Could you check a few things on this model? Use its own coordinates, in mm. Face numbers are marked on the shaded views. A direction names the side the tool comes from. Give positions to 0.01 mm unless a question says otherwise; leave off trailing zeros. Order: outer loops, then holes, each group sorted by start corner. A loop starts at its lowest first (then second) coordinate and runs counter-clockwise, first axis right, second up. Notation, with made-up numbers: M 41,-6 L 69,-6 A28 ccw 69,22 Z; hole C -6.5,-36.5 d3. An arc over 180 degrees is marked long. Use a Markdown table: item, result. Add a question column.
Item 1: Suppose I cut it at C-C on z = 37. Write out the boundary of the cut face in (x, y), plus the area to 3 significant figures.
Item 2: If we mould it in two halves opening along Z, with no side actions, what happens to the marked faces 3, 4 and 5? For each: released by +Z, released by -Z, zero draft, split by the parting line, or undercut.
Item 3: Suppose I cut it at B-B on y = 15. Write out the boundary of the cut face in (x, z), plus the area to 3 significant figures.
Item 4: If I drill on L1, parallel to Z at x = 46.5, y = 12.5; L2, parallel to X at y = 3.5, z = 52; L3, parallel to X at y = 7.5, z = 57.5, over which ranges is the centre line in solid material (lowest first)? Write a range as from..to.
Item 5: Suppose I cut it at A-A on x = 20. Write out the boundary of the cut face in (y, z).
Item 6: For the marked faces 1 and 2, which set-ups out of +Z, -Z, +X, -X, +Y, -Y let a thin tool reach every point of the face, with its end or its side?
Item 7: I'm going to push a flat-ended pin straight in: pin 1 Ø6 at (y, z) = (5, 29.5) entering from +X. Where does the tip first touch, or does it pass through?
from build123d import *

# Parameters (mm, degrees)
BOX_W        = 60
BOX_H        = 20
BOX_DEPTH    = 15
BOX001_W     = 15
BOX001_H     = 20
BOX001_DEPTH = 70
BOX002_W     = 60
BOX002_H     = 20
BOX002_DEPTH = 15
FILLET_R     = 5


with BuildPart() as cube:
    # Box → Box (new body)
    with BuildSketch(Plane.XY):
        with Locations((30, 10)):
            Rectangle(BOX_W, BOX_H)
    extrude(amount=BOX_DEPTH)


with BuildPart() as cube001:
    # Box001 → Box001 (new body)
    with BuildSketch(Plane.XY):
        with Locations((7.5, 10)):
            Rectangle(BOX001_W, BOX001_H)
    extrude(amount=BOX001_DEPTH)


with BuildPart() as fillet_body:
    # Box002 → Box002 (new body)
    with BuildSketch(Plane.XY.offset(55)):
        with Locations((30, 10)):
            Rectangle(BOX002_W, BOX002_H)
    extrude(amount=BOX002_DEPTH)

    # Fusion: union Cube, Cube001
    add(cube.part)
    add(cube001.part)

    # Fillet
    fillet_edges = [fillet_body.edges().sort_by_distance(p)[0] for p in [
        (0, 10, 70),
        (60, 10, 70),
        (0, 10, 0),
        (60, 10, 55),
        (60, 10, 15),
        (60, 10, 0),
    ]]
    fillet(fillet_edges, radius=FILLET_R)


solid = fillet_body.part
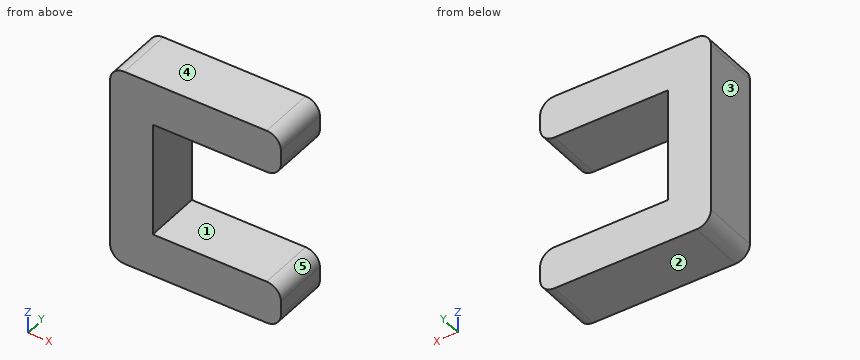
Findings below:
| question | item | result |
|---|---|---|
| 1 | outline | M 0,0 L 15,0 L 15,20 L 0,20 Z |
| 1 | area | 300 mm^2 |
| 2 | face 3 | zero draft |
| 2 | face 4 | released by +Z |
| 2 | face 5 | undercut |
| 3 | outline | M 0,5 A5 ccw 5,0 L 55,0 A5 ccw 60,5 L 60,10 A5 ccw 55,15 L 15,15 L 15,55 L 55,55 A5 ccw 60,60 L 60,65 A5 ccw 55,70 L 5,70 A5 ccw 0,65 Z |
| 3 | area | 2,370 mm^2 |
| 4 | L1 | z = 0..15, 55..70 |
| 4 | L2 | x = 0..15 |
| 4 | L3 | x = 0..59.33 |
| 5 | outline | M 0,0 L 20,0 L 20,15 L 0,15 Z; M 0,55 L 20,55 L 20,70 L 0,70 Z |
| 6 | face 1 | +X, +Y, -Y |
| 6 | face 2 | -Z, +X, -X, +Y, -Y |
| 7 | pin 1 | stops at x = 15 |
